```python
from build123d import *

# Parameters (mm, degrees)
SKETCH1_W                   = 30.95625
SKETCH1_H                   = 88.9
BOSS_EXTRUDE1_DEPTH         = 4.7625
FILLET1_R                   = 6.35
SKETCH6_R                   = 1.524
CUT_EXTRUDE1_DEPTH          = 5.7625
SKETCH7_R                   = 2.38125
CUT_EXTRUDE2_DEPTH          = 5.7625
BOSS_EXTRUDE3_DEPTH         = 1.524
F_4_40_TAPPED_HOLE1_D       = 2.2606
SKETCH10_R                  = 1.524
CUT_EXTRUDE3_DEPTH          = 2.524
SKETCH11_R                  = 3.175
CUT_EXTRUDE4_DEPTH          = 3.302
F_1_2_13_TAPPED_HOLE2_D     = 10.71626
F_1_2_13_TAPPED_HOLE2_DEPTH = 2.794
F_1_2_13_TAPPED_HOLE2_TIP   = 3.219489309


with BuildPart() as part:
    # Sketch1 → Boss-Extrude1 (new body)
    with BuildSketch(Plane(origin=(0, 0, 0), x_dir=(1, 0, 0), z_dir=(0, 1, 0))):
        Rectangle(SKETCH1_W, SKETCH1_H)
    extrude(amount=BOSS_EXTRUDE1_DEPTH)

    # Fillet1
    fillet1_edges = [part.edges().sort_by_distance(p)[0] for p in [
        (15.478125, 2.38125, -44.45),
        (15.478125, 2.38125, 44.45),
        (-15.478125, 2.38125, 44.45),
        (-15.478125, 2.38125, -44.45),
    ]]
    fillet(fillet1_edges, radius=FILLET1_R)

    # Sketch6 → Cut-Extrude1 (cut, through all)
    with BuildSketch(Plane.XZ):
        with Locations((0, 14.478)):
            Circle(SKETCH6_R)
        with Locations((0, -14.478)):
            Circle(SKETCH6_R)
    extrude(amount=-CUT_EXTRUDE1_DEPTH, mode=Mode.SUBTRACT)

    # Sketch7 → Cut-Extrude2 (cut, through all)
    with BuildSketch(Plane.XZ):
        with Locations((0, -39.116)):
            Circle(SKETCH7_R)
        with Locations((0, 39.116)):
            Circle(SKETCH7_R)
    extrude(amount=-CUT_EXTRUDE2_DEPTH, mode=Mode.SUBTRACT)

    # Sketch9 → Boss-Extrude3 (add)
    with BuildSketch(Plane.XZ):
        with BuildLine():
            Line((9.128125, -44.45), (-9.128125, -44.45))
            ThreePointArc((-9.128125, -44.45), (-13.618253061, -42.590128061), (-15.478125, -38.1))
            Line((-15.478125, -38.1), (-15.478125, 38.1))
            ThreePointArc((-15.478125, 38.1), (-13.618253061, 42.590128061), (-9.128125, 44.45))
            Line((-9.128125, 44.45), (9.128125, 44.45))
            ThreePointArc((9.128125, 44.45), (13.618253061, 42.590128061), (15.478125, 38.1))
            Line((15.478125, 38.1), (15.478125, -38.1))
            ThreePointArc((15.478125, -38.1), (13.618253061, -42.590128061), (9.128125, -44.45))
        make_face()
    extrude(amount=BOSS_EXTRUDE3_DEPTH)

    # #4-40 Tapped Hole1 (through all)
    with Locations(Plane(origin=(0, 4.7625, 0), x_dir=(-1, 0, 0), z_dir=(0, 1, 0))):
        with Locations((0, 25.4), (0, -25.4)):
            Hole(F_4_40_TAPPED_HOLE1_D / 2)

    # Sketch10 → Cut-Extrude3 (cut, through all)
    with BuildSketch(Plane(origin=(0, 0, 0), x_dir=(1, 0, 0), z_dir=(0, 1, 0))):
        with Locations((0, -14.478)):
            Circle(SKETCH10_R)
        with Locations((0, 14.478)):
            Circle(SKETCH10_R)
    extrude(amount=-CUT_EXTRUDE3_DEPTH, mode=Mode.SUBTRACT)

    # Sketch11 → Cut-Extrude4 (cut)
    with BuildSketch(Plane.XZ.offset(1.524)):
        with Locations((0, -14.478)):
            Circle(SKETCH11_R)
        with Locations((0, 14.478)):
            Circle(SKETCH11_R)
    extrude(amount=-CUT_EXTRUDE4_DEPTH, mode=Mode.SUBTRACT)

    # 1/2-13 Tapped Hole2
    with Locations(Plane(origin=(0, 4.7625, 0), x_dir=(-1, 0, 0), z_dir=(0, 1, 0))):
        with Locations((0, 0)):
            Hole(F_1_2_13_TAPPED_HOLE2_D / 2, depth=F_1_2_13_TAPPED_HOLE2_DEPTH)
            with Locations((0, 0, -(F_1_2_13_TAPPED_HOLE2_DEPTH + F_1_2_13_TAPPED_HOLE2_TIP / 2))):  # 118° drill point
                Cone(0, F_1_2_13_TAPPED_HOLE2_D / 2, F_1_2_13_TAPPED_HOLE2_TIP, mode=Mode.SUBTRACT)


solid = part.part
```
The listing builds one solid part. Answer for the finished solid, in the listing's coordinates (mm). A direction names the side the tool comes from. Coordinates: 2 decimals unless noted, no trailing zeros. Loops run counter-clockwise (first coordinate to the right, second up) from the corner with the lowest first, then second, coordinate; pieces in that order, holes last. Notation, with made-up numbers: (-8.5, 84) - (25.5, 84) arc R28 cw to (25.5, 106) - close; hole circle Ø11 at (44.5, 11). An arc over 180 degrees is marked (long way). Write item = value, one per line.
1) Determine the mould class of faces 1 (the face through (0, 2, -44.45)), 2 (the face through (-0.198, 3.291, 12.967)), 3 (the face through (0, 2, 44.45)) for opening direction Z: pulls with the +Z half, pulls with the -Z half, needs draft (parallel to the pull), parting line crosses it, or undercut.
Responses:
face_1 = pulls with the -Z half
face_2 = undercut
face_3 = pulls with the +Z half
2) Find the intervals of material crossed by line 1 along X through (y, z) = (2.85, 0); line 2 along X through (y, z) = (0.5, 14.5); line 3 along Z through (x, y) = (-3.5, 3.25), in increasing order.
Responses:
line_1 = -15.48 to -5.36, 5.36 to 15.48
line_2 = -15.48 to -3.17, 3.17 to 15.48
line_3 = -44.45 to -4.06, 4.06 to 44.45
3) Section A-A (z = -25.4) is taken. Determine the outline of the cut face in (x, y).
Responses:
outline = (-15.48, -1.52) - (-1.13, -1.52) - (-1.13, 4.76) - (-15.48, 4.76) - close; (1.13, -1.52) - (15.48, -1.52) - (15.48, 4.76) - (1.13, 4.76) - close
4) Which of the six approach directions +Z, -Z, +X, -X, +Y, -Y give full straight-line access (tool end or side, diameter ignored) to faces 4 (the face through (-0.33, 3.29, -12.99)), 5 (the face through (1.707, 0.104, 17.155)), 6 (the face through (2.472, 3.346, -4.754))?
Responses:
face_4 = +Y, -Y
face_5 = -Y
face_6 = +Y
5) Each of these flat-tipped pins is pushed along its axis until it touches: P1, Ø8.5, axis at x = 0, z = 14.478, coming from the -Y side; P2, Ø4, axis at x = 0, z = -39.116, coming from the +Y side; P3, Ø3, axis at x = -0.5, z = 16, coming from the -Y side. Where does it stop, or does it pass through?
Responses:
P1 = -1.52
P2 = 0
P3 = 1.78
6) Section B-B (y = 3.5) is taken. Determine the outline of the cut face in (x, z), plus the area to 3 significant figures.
Responses:
outline = (-15.48, -38.1) arc R6.35 ccw to (-9.13, -44.45) - (9.13, -44.45) arc R6.35 ccw to (15.48, -38.1) - (15.48, 38.1) arc R6.35 ccw to (9.13, 44.45) - (-9.13, 44.45) arc R6.35 ccw to (-15.48, 38.1) - close; hole circle Ø10.72 at (0, 0); hole circle Ø4.76 at (0, -39.12); hole circle Ø4.76 at (0, 39.12); hole circle Ø3.05 at (0, -14.48); hole circle Ø3.05 at (0, 14.48); hole circle Ø2.26 at (0, -25.4); hole circle Ø2.26 at (0, 25.4)
area = 2,570 mm^2
